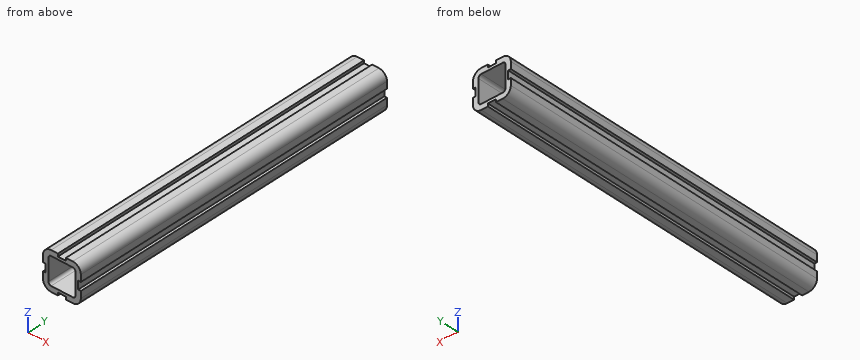
Autodesk Inventor part; units mm, degrees
ref_plane "Start Plane" through (0, 28, 0) normal (0, 1, 0) x (-1, 0, 0)
ref_plane "End Plane" through (0, 276.8, 0) normal (0, 1, 0) x (-1, 0, 0)
ref_plane "Work Plane4" through (-290.8, 28, -8) normal (0, -1, 0) x (1, 0, 0)
ref_plane "Start Plane" through (0, 28, 0) normal (0, 1, 0) x (-1, 0, 0)
ref_plane "End Plane" through (0, 276.8, 0) normal (0, 1, 0) x (-1, 0, 0)
sketch "Sketch" plane through (0, 0, 0) normal (0, 1, 0) x (-1, 0, 0)
  line L0 (8, -10) -> (-8, -10)
  line L1 (-10, -8) -> (-10, 8)
  line L2 (-8, 10) -> (8, 10)
  line L3 (10, 8) -> (10, -8)
  line L4 (10, -10) -> (-10, 10) construction
  line L5 (-10, -10) -> (10, 10) construction
  line L6 (14, -14) -> (-14, 14) construction
  line L7 (-14, -14) -> (14, 14) construction
  arc A0 (8, -10) -> (10, -8) centre (8, -8) ccw
  arc A1 (-10, -8) -> (-8, -10) centre (-8, -8) ccw
  arc A2 (-8, 10) -> (-10, 8) centre (-8, 8) ccw
  arc A3 (10, 8) -> (8, 10) centre (8, 8) ccw
  arc A4 (8, -14) -> (14, -8) centre (8, -8) ccw
  arc A5 (-14, -8) -> (-8, -14) centre (-8, -8) ccw
  arc A6 (-8, 14) -> (-14, 8) centre (-8, 8) ccw
  arc A7 (14, 8) -> (8, 14) centre (8, 8) ccw
  line L8 (3, -14) -> (3, -12)
  line L9 (3, -12) -> (-3, -12)
  line L10 (-3, -12) -> (-3, -14)
  line L11 (-14, -3) -> (-12, -3)
  line L12 (-12, -3) -> (-12, 3)
  line L13 (-12, 3) -> (-14, 3)
  line L14 (-3, 14) -> (-3, 12)
  line L15 (-3, 12) -> (3, 12)
  line L16 (3, 12) -> (3, 14)
  line L17 (14, 3) -> (12, 3)
  line L18 (12, 3) -> (12, -3)
  line L19 (12, -3) -> (14, -3)
  line L20 (0, -10) -> (0, -12) construction
  line L21 (-10, 0) -> (-12, 0) construction
  line L22 (0, 10) -> (0, 12) construction
  line L23 (10, 0) -> (12, 0) construction
  line L24 (14, 8) -> (14, 3)
  line L25 (14, -3) -> (14, -8)
  line L26 (8, -14) -> (3, -14)
  line L27 (-3, -14) -> (-8, -14)
  line L28 (-14, -8) -> (-14, -3)
  line L29 (-14, 3) -> (-14, 8)
  line L30 (-8, 14) -> (-3, 14)
  line L31 (3, 14) -> (8, 14)
  point P0 (0, 0)
  dimension "d1" = 20
  dimension "d2" = 2
  dimension "d3" = 6
  dimension "d4" = 20
  dimension "d5" = 6
  dimension "d6" = 2
  dimension "d8" = 28
extrude "Body" add sketch "Sketch" along normal up to surface (248.8 mm away) from surface at 28
sketch "Sketch2" plane through (0, 0, 0) normal (0, 1, 0) x (-1, 0, 0)
  line L0 (0, 0) -> (10, 0)
ref_plane "Work Plane3" through (0, 0, 0) normal (0, 0, -1) x (-1, 0, 0)
sketch "Sketch3" plane through (0, 0, 0) normal (0, 0, -1) x (-1, 0, 0)
  line L0 (-2, 28) -> (12, 28) construction
  line L1 (-2, 276.8) -> (12, 276.8) construction
  dimension "d16" = 248.8
ref_plane "Work Plane4" through (-290.8, 28, -8) normal (0, -1, 0) x (1, 0, 0)
split "Split1" plane through (-290.8, 28, -8) removes the side toward (0, -1, 0)
ref_plane "Work Plane5" through (14, 276.8, -8) normal (0, 1, 0) x (1, 0, 0)
split "Split2" plane through (14, 276.8, -8) removes the side toward (0, 1, 0)
equation "\"G_OFFSET_START\" = -28"
equation "\"G_OFFSET_END\" = -28"
equation "\"d11\" = -G_OFFSET_START"
equation "\"d12\" = Length + G_OFFSET_END"
equation "\"G_L\" = d16"
properties part number "CE-5.2.2-PR" material "Steel, Mild"
Check sheet for the modelled part. Datum: model origin and axes. Units: mm. Coordinates: 2 decimals unless noted, no trailing zeros. Write each loop counter-clockwise with the first axis right and the second up, starting at its lowest first coordinate (ties: lowest second). Pieces come first, ordered by that corner, then holes. Notation, with made-up numbers: (9.5, 70.25) - (67.5, 70.25) arc R11 ccw to (67.5, 75.25) - close; hole circle Ø9 at (23, -11). An arc over 180 degrees is marked (long way). One line per question, with ' | ' between items.
Item 1: Sectioned sample at A-A on x = -0.5. Record the boundary of the cut face in (y, z).
Determined:
outline: (28, -12) - (276.8, -12) - (276.8, -10) - (28, -10) - close; (28, 10) - (276.8, 10) - (276.8, 12) - (28, 12) - close
Item 2: Thickness scan on line 1 (Z direction, x = 8.25, y = 144); line 2 (X direction, y = 262, z = -12.5); line 3 (X direction, y = 62, z = -2.75). Record the ranges inside material, lowest first. Write a range as [from, to].
Determined:
line 1: z = [-13.99, -9.98], [9.98, 13.99] | line 2: x = [-11.97, -3], [3, 11.97] | line 3: x = [-12, -10], [10, 12]
Item 3: Gauge pin test, flat ends, axial feed: P1, Ø2, axis at y = 144.5, z = -12.5, coming from the +X side; P2, Ø2, axis at x = -13, y = 162, coming from the -Z side; P3, Ø1, axis at y = 108, z = 13.5, coming from the -X side. Record the tip position at first contact, or that the pin passes through.
Determined:
P1: stops at x = 12.87 | P2: stops at z = -12.47 | P3: stops at x = -11.32
